Design review of the part built by this model. Coordinates are the model's own, in mm. Give positions to 0.01 mm unless a question says otherwise; leave off trailing zeros. Order: outer loops, then holes, each group sorted by start corner. A loop starts at its lowest first (then second) coordinate and runs counter-clockwise, first axis right, second up. Notation, with made-up numbers: M 54,87 L 93,87 A23 ccw 93,104 Z; hole C 57.5,73 d3. An arc over 180 degrees is marked long. Answer as a JSON object with one key per item and string values.
Autodesk Inventor part; units mm, degrees
ref_plane "YZ Plane" through (0, 0, 0) normal (1, 0, 0) x (0, 1, 0)
ref_plane "XZ Plane" through (0, 0, 0) normal (0, 1, 0) x (-1, 0, 0)
ref_plane "XY Plane" through (0, 0, 0) normal (0, 0, 1) x (1, 0, 0)
sketch "Sketch1" plane through (0, 0, 0) normal (1, 0, 0) x (0, 1, 0)
  line L0 (0, 80.3974) -> (25.4, 80.3974)
  line L1 (25.4, 80.3974) -> (25.4, -97.4026)
  line L2 (25.4, -97.4026) -> (0, -97.4026)
  line L3 (0, -97.4026) -> (0, 80.3974)
  point P0 (0, 0)
  dimension "d0" = 177.8
  dimension "d1" = 25.4
  dimension "d2" = 0
extrude "Extrusion1" add sketch "Sketch1" along normal blind 2.921
sketch "Sketch2" plane through (2.921, 0, 0) normal (1, 0, 0) x (0, 0, -1)
  line L0 (-80.3974, 0) -> (97.4026, 0)
  line L1 (-67.6974, 0) -> (-54.9974, 0)
  line L2 (-54.9974, 0) -> (-54.9974, 2.921)
  line L3 (-54.9974, 2.921) -> (-67.6974, 2.921)
  line L4 (-67.6974, 2.921) -> (-67.6974, 0)
  line L5 (-80.3974, 25.4) -> (-80.3974, 0)
  line L6 (-42.2974, 0) -> (-29.5974, 0)
  line L7 (-29.5974, 0) -> (-29.5974, 2.921)
  line L8 (-29.5974, 2.921) -> (-42.2974, 2.921)
  line L9 (-42.2974, 2.921) -> (-42.2974, 0)
  line L10 (-16.8974, 0) -> (-4.1974, 0)
  line L11 (-4.1974, 0) -> (-4.1974, 2.921)
  line L12 (-4.1974, 2.921) -> (-16.8974, 2.921)
  line L13 (-16.8974, 2.921) -> (-16.8974, 0)
  line L14 (8.5026, 0) -> (21.2026, 0)
  line L15 (21.2026, 0) -> (21.2026, 2.921)
  line L16 (21.2026, 2.921) -> (8.5026, 2.921)
  line L17 (8.5026, 2.921) -> (8.5026, 0)
  line L18 (33.9026, 0) -> (46.6026, 0)
  line L19 (46.6026, 0) -> (46.6026, 2.921)
  line L20 (46.6026, 2.921) -> (33.9026, 2.921)
  line L21 (33.9026, 2.921) -> (33.9026, 0)
  line L22 (59.3026, 0) -> (72.0026, 0)
  line L23 (72.0026, 0) -> (72.0026, 2.921)
  line L24 (72.0026, 2.921) -> (59.3026, 2.921)
  line L25 (59.3026, 2.921) -> (59.3026, 0)
  line L26 (84.7026, 0) -> (97.4026, 0)
  line L27 (97.4026, 0) -> (97.4026, 2.921)
  line L28 (97.4026, 2.921) -> (84.7026, 2.921)
  line L29 (84.7026, 2.921) -> (84.7026, 0)
  point P0 (0, 0)
  dimension "d5" = 12.7
  dimension "d6" = 2.921
  dimension "d7" = 12.7
  dimension "d10" = 25.4
extrude "Extrusion2" cut sketch "Sketch2" against normal blind 2.921
sketch "Sketch3" plane through (2.921, 0, 0) normal (1, 0, 0) x (0, 0, -1)
  line L0 (-67.6974, 2.921) -> (-67.6974, 0)
  line L1 (-80.3974, 25.4) -> (-80.3974, 0)
  line L2 (-67.6974, 2.921) -> (-80.3974, 2.921)
  line L3 (-80.3974, 2.921) -> (-80.3974, 0)
  line L4 (-80.3974, 0) -> (-67.6974, 0)
  line L5 (-67.6974, 0) -> (-67.6974, 2.921)
  point P0 (0, 0)
extrude "Extrusion3" cut sketch "Sketch3" against normal blind 25.4
sketch "Sketch4" plane through (0, 0, 16.8974) normal (0, -1, 0) x (1, 0, 0)
  line L0 (2.921, 12.7) -> (0, 12.7)
  line L1 (0, 0) -> (0, 12.7)
  line L2 (0, 0) -> (2.921, 0)
  line L3 (2.921, 12.7) -> (2.921, 0)
  point P0 (0, -16.8974)
extrude "Extrusion4" add sketch "Sketch4" along normal blind 38.1
fillet "Fillet1" radius 6.35 2 edges at (1.4605, -38.1, 29.5974) (1.4605, -38.1, 16.8974)
sketch "Sketch5" plane through (2.921, 0, 0) normal (1, 0, 0) x (0, 0, -1)
  line L0 (-21.754, -28.8443) -> (-26.6184, -32.926)
  line L1 (-26.6184, -32.926) -> (-24.7408, -35.1637)
  line L2 (-24.7408, -35.1637) -> (-19.8764, -31.082)
  line L3 (-19.8764, -31.082) -> (-21.754, -28.8443)
  line L4 (-21.754, -28.8443) -> (-24.7408, -35.1637) construction
  line L5 (-26.6184, -32.926) -> (-19.8764, -31.082) construction
  line L6 (-16.8974, 2.921) -> (-16.8974, -31.75)
  line L7 (-16.8974, 2.921) -> (-4.1974, 2.921)
  point P0 (0, 0)
  point P1 (-23.2474, -32.004)
  dimension "d22" = 6.35
  dimension "d23" = 2.921
  dimension "d24" = 6.35
  dimension "d25" = 34.925
  dimension "d29" = 40
extrude "Extrusion5" cut sketch "Sketch5" against normal blind 38.1
sketch "Sketch6" plane through (0, 0, 0) normal (-1, 0, 0) x (0, 0, 1)
  circle A0 centre (67.6974, 12.7) radius 1.5875
  circle A1 centre (54.9974, 12.7) radius 1.5875
  line L0 (80.3974, 25.4) -> (-97.4026, 25.4)
  line L1 (80.3974, 2.921) -> (80.3974, 25.4)
  point P0 (0, 0)
  dimension "d30" = 3.175
  dimension "d31" = 3.175
  dimension "d32" = 12.7
  dimension "d33" = 12.7
  dimension "d34" = 12.7
  dimension "d35" = 12.7
extrude "Extrusion6" cut sketch "Sketch6" against normal blind 38.1
fillet "Fillet2" radius 6.35 2 edges at (1.4605, 25.4, -97.4026) (1.4605, 25.4, 80.3974)
sketch "Sketch7" plane through (2.921, 0, 0) normal (1, 0, 0) x (0, 0, -1)
  line L0 (59.3026, 2.921) -> (72.0026, 2.921)
  line L1 (72.0026, 2.921) -> (72.0026, 13.081)
  line L2 (72.0026, 13.081) -> (59.3026, 13.081)
  line L3 (59.3026, 13.081) -> (59.3026, 2.921)
  point P0 (0, 0)
  dimension "d39" = 12.7
  dimension "d40" = 10.16
extrude "Extrusion7" cut sketch "Sketch7" against normal blind 25.4
sketch "Sketch9" plane through (2.921, 0, 0) normal (1, 0, 0) x (0, 0, -1)
  line L0 (56.1276, 15.24) -> (43.4276, 15.24)
  line L1 (43.4276, 15.24) -> (43.4276, 5.08)
  line L2 (43.4276, 5.08) -> (56.1276, 5.08)
  line L3 (56.1276, 5.08) -> (56.1276, 15.24)
  line L4 (59.3026, 0) -> (59.3026, 13.081)
  line L5 (97.4026, 2.921) -> (97.4026, 19.05)
  line L6 (46.6026, 0) -> (59.3026, 0)
  point P0 (0, 0)
  dimension "d43" = 3.175
  dimension "d44" = 53.975
  dimension "d45" = 10.16
  dimension "d46" = 5.08
extrude "Extrusion8" cut sketch "Sketch9" against normal blind 25.4
properties part number "wall"
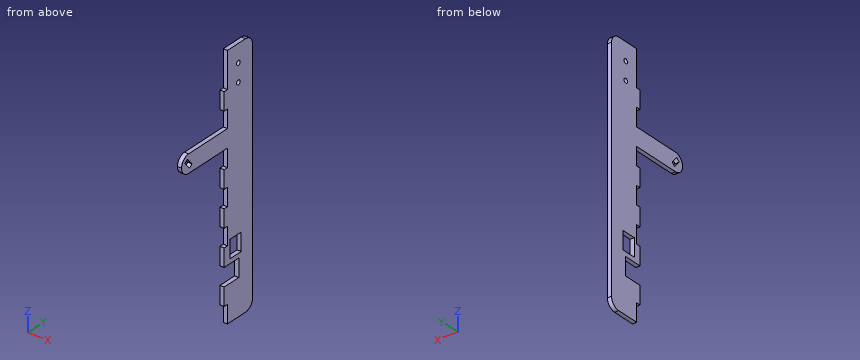
(1) We need section A-A (x = 2.4). Count the separate pieces of the cut face and the enclosed holes in it, plus the area to 3 significant figures.
Checked values:
{"separate pieces": "1", "enclosed holes": "4", "area": "4,380 mm^2"}
(2) To check wall thickness, follow L1, parallel to Z at x = 1.7, y = 2; L2, parallel to Z at x = 1.5, y = 7.5; L3, parallel to Y at x = 1.9, z = -8. State the ranges of each line that lie inside material, in increasing order. Write a range as from..to.
Checked values:
{"L1": "z = -84.7..-72, -59.3..-46.6, -33.9..-21.2, -8.5..4.2, 16.9..29.6, 42.3..55", "L2": "z = -97.4..-72, -59.3..-56.13, -43.43..80.4", "L3": "y = 0..25.4"}
(3) Insertion check: pin 1 (1.5 mm diameter, centred on x = 1, y = 1, fed in from +Z); pin 2 (0.9 mm diameter, centred on x = 1.5, z = -17.5, fed in from -Y); pin 3 (1 mm diameter, centred on x = 2, y = -5, fed in from +Z); pin 4 (3 mm diameter, centred on y = 12.7, z = 55, fed in from -X). Each pin has a flat end and moves straight along its axis. Give the tip position at first contact, or say it passes through.
Checked values:
{"pin 1": "stops at z = 55", "pin 2": "stops at y = 2.92", "pin 3": "stops at z = 29.6", "pin 4": "passes through"}
(4) We need section B-B (y = -4). Write out the cut boundary in (x, z).
Checked values:
{"outline": "M 0,16.9 L 2.92,16.9 L 2.92,29.6 L 0,29.6 Z"}
